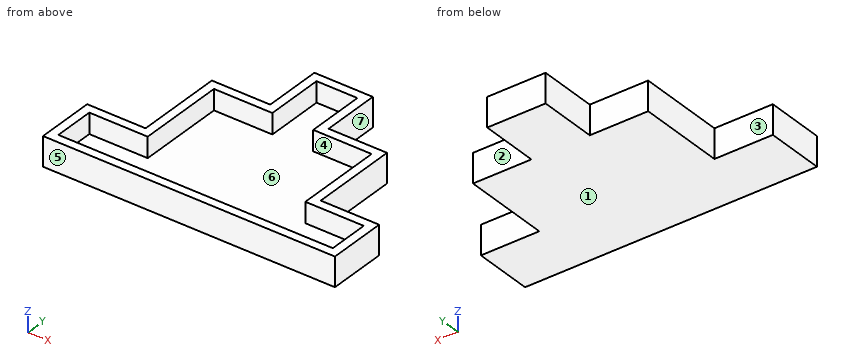
```python
from build123d import *

# Parameters (mm, degrees)
BOSS_EXTRUDE1_DEPTH = 15
BOSS_EXTRUDE2_DEPTH = 4.5


with BuildPart() as part:
    # Sketch1 → Boss-Extrude1 (new body)
    with BuildSketch(Plane.XY):
        Polygon((75, 0), (-75, 0), (-75, 30), (-45, 30), (-45, 75), (-15, 75), (-15, 105), (15, 105), (15, 75), (45, 75), (45, 30), (75, 30), align=None)
        Polygon((-70.5, 4.5), (-70.5, 25.5), (-40.5, 25.5), (-40.5, 70.5), (-10.5, 70.5), (-10.5, 100.5), (10.5, 100.5), (10.5, 70.5), (40.5, 70.5), (40.5, 25.5), (70.5, 25.5), (70.5, 4.5), align=None, mode=Mode.SUBTRACT)
    extrude(amount=BOSS_EXTRUDE1_DEPTH)

    # Sketch1<2> → Boss-Extrude2 (add)
    with BuildSketch(Plane.XY):
        Polygon((-70.5, 4.5), (-70.5, 25.5), (-40.5, 25.5), (-40.5, 70.5), (-10.5, 70.5), (-10.5, 100.5), (10.5, 100.5), (10.5, 70.5), (40.5, 70.5), (40.5, 25.5), (70.5, 25.5), (70.5, 4.5), align=None)
    extrude(amount=BOSS_EXTRUDE2_DEPTH)


solid = part.part
```
Model file for the job. Use its own axes, mm. Face numbers are marked on the shaded views. A direction names the side the tool comes from. Coordinates: 2 decimals unless noted, no trailing zeros. Order: outer loops, then holes, each group sorted by start corner. A loop starts at its lowest first (then second) coordinate and runs counter-clockwise, first axis right, second up. Notation, with made-up numbers: (71, -24.75) -> (98, -24.75) arc R24 cw to (98, -1.75) -> close; hole circle Ø9 at (43, 59). An arc over 180 degrees is marked (long way). Return JSON: item names as keys, results as strings.
Item 1: Mould opens along X. For the marked faces 5, 6 and 7 say: pulls with the +X half, pulls with the -X half, needs draft (parallel to the pull), parting line crosses it, or undercut.
Model answer:
{"face 5": "needs draft", "face 6": "undercut", "face 7": "pulls with the +X half"}
Item 2: Slice it at D-D (z = 2.75). Write the cut outline in (x, y).
Model answer:
{"outline": "(-75, 0) -> (75, 0) -> (75, 30) -> (45, 30) -> (45, 75) -> (15, 75) -> (15, 105) -> (-15, 105) -> (-15, 75) -> (-45, 75) -> (-45, 30) -> (-75, 30) -> close"}
Item 3: Slice it at C-C (y = 62). Write the cut outline in (x, z).
Model answer:
{"outline": "(-45, 0) -> (45, 0) -> (45, 15) -> (40.5, 15) -> (40.5, 4.5) -> (-40.5, 4.5) -> (-40.5, 15) -> (-45, 15) -> close"}
Item 4: 3-axis set-ups, long thin cutter, end or side, ignore diameter. For the marked faces 1, 2, 3 and 4: which of +Z, -Z, +X, -X, +Y, -Y reach the whole face in a straight line?
Model answer:
{"face 1": "-Z, +X, -X, +Y, -Y", "face 2": "+Z, -Z, +X, +Y", "face 3": "+Z, -Z, -X, +Y", "face 4": "+Z"}
Item 5: Slice it at B-B (z = 11.5). Write the cut outline in (x, y), then the cut area to 3 significant figures.
Model answer:
{"outline": "(-75, 0) -> (75, 0) -> (75, 30) -> (45, 30) -> (45, 75) -> (15, 75) -> (15, 105) -> (-15, 105) -> (-15, 75) -> (-45, 75) -> (-45, 30) -> (-75, 30) -> close; hole (-70.5, 4.5) -> (70.5, 4.5) -> (70.5, 25.5) -> (40.5, 25.5) -> (40.5, 70.5) -> (10.5, 70.5) -> (10.5, 100.5) -> (-10.5, 100.5) -> (-10.5, 70.5) -> (-40.5, 70.5) -> (-40.5, 25.5) -> (-70.5, 25.5) -> close", "area": "2,210 mm²"}
Item 6: Wall check: line 1 along X through (y, z) = (44, 8.5); line 2 along Y through (x, z) = (-64, 6.25); line 3 along Y through (x, z) = (44.5, 8.25). Give the ranges that are in metal, low to high. Write a range as from..to.
Model answer:
{"line 1": "x = -45..-40.5, 40.5..45", "line 2": "y = 0..4.5, 25.5..30", "line 3": "y = 0..4.5, 25.5..75"}
Item 7: Pin check, flat tips, straight feed: P1, Ø1, axis at y = 71, z = 6, coming from the -X side; P2, Ø4.5, axis at x = 60, z = 9, coming from the +Y side; P3, Ø3, axis at x = -2, z = 7.5, coming from the -Y side; P4, Ø7.5, axis at x = -25, z = 8.5, coming from the +Y side. Stop position of each tip, or through.
Model answer:
{"P1": "stops at x = -45", "P2": "stops at y = 30", "P3": "stops at y = 0", "P4": "stops at y = 75"}
Item 8: Slice it at A-A (x = 6). Write the cut outline in (y, z), then the cut area to 3 significant figures.
Model answer:
{"outline": "(0, 0) -> (105, 0) -> (105, 15) -> (100.5, 15) -> (100.5, 4.5) -> (4.5, 4.5) -> (4.5, 15) -> (0, 15) -> close", "area": "567 mm²"}
